Check sheet for the modelled part. Datum: model origin and axes. Units: mm. Face numbers are marked on the shaded views. A direction names the side the tool comes from. Give positions to 0.01 mm unless a question says otherwise; leave off trailing zeros. Write each loop counter-clockwise with the first axis right and the second up, starting at its lowest first coordinate (ties: lowest second). Pieces come first, ordered by that corner, then holes. Notation, with made-up numbers: M 61,-2 L 102,-2 A23 cw 102,32 Z; hole C 45.5,21.25 d7. An arc over 180 degrees is marked long. Write each question's results on one line, items separated by ' | '. Start each with the question number.
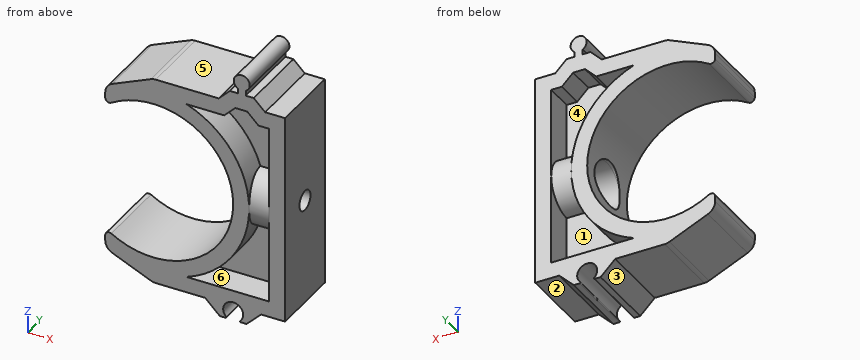
from build123d import *

# Parameters (mm, degrees)
BOSS_EXTRUDE1_DEPTH = 18
CUT_EXTRUDE1_DEPTH  = 7
BOSS_EXTRUDE2_DEPTH = 7
SKETCH4_R           = 2.5
CUT_EXTRUDE2_DEPTH  = 6
SKETCH5_R           = 5.75
CUT_EXTRUDE3_DEPTH  = 7
CUT_EXTRUDE4_START  = -7
SKETCH6_R           = 5.75
CUT_EXTRUDE4_DEPTH  = 7


with BuildPart() as part:
    # Sketch1 → Boss-Extrude1 (new body)
    with BuildSketch(Plane(origin=(0, 0, 0), x_dir=(1, 0, 0), z_dir=(0, 1, 0))):
        with BuildLine():
            Line((10.653013329, -29.309744988), (10.653013329, -30.57769418))
            ThreePointArc((10.653013329, -30.57769418), (11.653013329, -34.309744988), (12.653013329, -30.57769418))
            Line((12.653013329, -30.57769418), (12.653013329, -29.309744988))
            Line((12.653013329, -29.309744988), (14.653013329, -29.309744988))
            Line((14.653013329, -29.309744988), (17.5, -26.5))
            Line((17.5, -26.5), (22.5, -26.5))
            Line((22.5, -26.5), (22.5, 26.5))
            Line((22.5, 26.5), (16.5, 26.5))
            Line((16.5, 26.5), (12.844502727, 30.107679392))
            Line((12.844502727, 30.107679392), (11.410696035, 30.107679392))
            ThreePointArc((11.410696035, 30.107679392), (11.225950376, 29.984289062), (11.269162996, 29.766369807))
            ThreePointArc((11.269162996, 29.766369807), (9.5, 25.5), (7.730837004, 29.766369807))
            ThreePointArc((7.730837004, 29.766369807), (7.774049624, 29.984289062), (7.589303965, 30.107679392))
            Line((7.589303965, 30.107679392), (6.155497273, 30.107679392))
            Line((6.155497273, 30.107679392), (2.5, 26.5))
            Line((2.5, 26.5), (-9.870833143, 26.5))
            ThreePointArc((-9.870833143, 26.5), (-10.486603861, 26.436124388), (-11.076152757, 26.247217616))
            Line((-11.076152757, 26.247217616), (-20.702456422, 22.023754373))
            Line((-20.702456422, 22.023754373), (-20.705319614, 22.022498171))
            ThreePointArc((-20.705319614, 22.022498171), (-22.011569115, 20.916018371), (-22.5, 19.275280555))
            Line((-22.5, 19.275280555), (-22.5, 17.88854382))
            ThreePointArc((-22.5, 17.88854382), (-21.987950036, 17.015672259), (-20.976190476, 17.0367084))
            ThreePointArc((-20.976190476, 17.0367084), (9.5, 0), (-20.976190476, -17.0367084))
            ThreePointArc((-20.976190476, -17.0367084), (-21.987950036, -17.015672259), (-22.5, -17.88854382))
            Line((-22.5, -17.88854382), (-22.5, -19.287953276))
            ThreePointArc((-22.5, -19.287953276), (-22.010713993, -20.929999331), (-20.702456502, -22.03642528))
            Line((-20.702456502, -22.03642528), (-11.074921132, -26.248472005))
            ThreePointArc((-11.074921132, -26.248472005), (-10.486705619, -26.43644479), (-9.87246463, -26.5))
            Line((-9.87246463, -26.5), (5.880022863, -26.5))
            Line((5.880022863, -26.5), (8.653013329, -29.309744988))
            Line((8.653013329, -29.309744988), (10.653013329, -29.309744988))
        make_face()
    extrude(amount=BOSS_EXTRUDE1_DEPTH)

    # Sketch2 → Cut-Extrude1 (cut)
    with BuildSketch(Plane.XZ):
        with BuildLine():
            Line((18.5, 22.5), (18.5, -22.5))
            Line((18.5, -22.5), (-2.148353456, -22.5))
            ThreePointArc((-2.148353456, -22.5), (13.5, 0), (-2.148353456, 22.5))
            Line((-2.148353456, 22.5), (7.238559187, 22.5))
            Line((7.238559187, 22.5), (10.039345887, 25.282038261))
            Line((10.039345887, 25.282038261), (13.039345883, 25.282178795))
            Line((13.039345883, 25.282178795), (15.843268341, 22.5))
            Line((15.843268341, 22.5), (18.5, 22.5))
        make_face()
    cut_extrude1 = extrude(amount=-CUT_EXTRUDE1_DEPTH, mode=Mode.SUBTRACT)

    # Mirror1: Cut-Extrude1 across plane
    add(cut_extrude1.mirror(Plane(origin=(0, 9, 0), x_dir=(0, 0, 1), z_dir=(0, -1, 0))), mode=Mode.SUBTRACT)

    # Sketch3 → Boss-Extrude2 (add)
    with BuildSketch(Plane.ZY.offset(-18.5)):
        with BuildLine():
            Line((7, 7), (-7, 7))
            ThreePointArc((-7, 7), (0, 0), (7, 7))
        make_face()
    boss_extrude2 = extrude(amount=BOSS_EXTRUDE2_DEPTH)

    # Mirror2: Boss-Extrude2 across plane
    add(boss_extrude2.mirror(Plane(origin=(0, 9, 0), x_dir=(0, 0, 1), z_dir=(0, -1, 0))))

    # Sketch4 → Cut-Extrude2 (cut)
    with BuildSketch(Plane(origin=(22.5, 0, 0), x_dir=(0, 0, -1), z_dir=(1, 0, 0))):
        with Locations((0, 9)):
            Circle(SKETCH4_R)
    extrude(amount=-CUT_EXTRUDE2_DEPTH, mode=Mode.SUBTRACT)

    # Sketch5 → Cut-Extrude3 (cut)
    with BuildSketch(Plane(origin=(9.5, 0, 0), x_dir=(0, 0, -1), z_dir=(1, 0, 0))):
        with Locations((0, 9)):
            Circle(SKETCH5_R)
    extrude(amount=-CUT_EXTRUDE3_DEPTH, mode=Mode.SUBTRACT)

    # Sketch6 → Cut-Extrude4 (cut)
    with BuildSketch(Plane.ZY.offset(-9.5).offset(CUT_EXTRUDE4_START)):
        with Locations(Location((0, 9, 0), (0, 0, 180))):
            Circle(SKETCH6_R)
    extrude(amount=CUT_EXTRUDE4_DEPTH, mode=Mode.SUBTRACT)


solid = part.part
Q1. Tool access check on the marked faces 4, 5 and 6. Record the directions out of +Z, -Z, +X, -X, +Y, -Y that give a thin tool (end or side, any length) a straight path to the whole face; none if there is none.
Q2. Scan lines: L1, parallel to Z at x = 10.5, y = 7.5; L2, parallel to Z at x = 10, y = 14; L3, parallel to Z at x = 6, y = 13.5. Record each from-to range of solid material in increasing order.
Q3. Depth check by flat-ended pin: pin 1 Ø4 at (x, y) = (2, 10.5) entering from -Z; pin 2 Ø2 at (y, z) = (6.5, -5.5) entering from -X; pin 3 Ø2 at (x, y) = (17, 4) entering from -Z. Enter the tip coordinate at first touch or a pass-through.
Q4. Section check A-A on x = 1. Record the boundary of the cut face in (y, z), plus the area to 3 significant figures.
Q5. Section check D-D on z = 10. Record the boundary of the cut face in (x, y), plus the area to 3 significant figures.
Q6. Release check for a two-part mould opening along X. For the marked faces 1, 2 and 3 record: pulls with the +X half, pulls with the -X half, needs draft (parallel to the pull), parting line crosses it, or undercut.
Q7. Section check C-C on y = 16. State how many separate pieces and enclosed holes the cut face has, plus the area to 3 significant figures.
Q8. Section check B-B on z = -12. Record the boundary of the cut face in (x, y), plus the area to 3 significant figures.
Check result:
1) face 4: +Y | face 5: +Z, -X, +Y, -Y | face 6: -Y
2) L1: -25.71 to -5.55, 5.55 to 29.31, 30.68 to 33.94 | L2: -25.55 to -22.5, -12.48 to -2.84, 2.84 to 12.48, 25.24 to 29.31, 31.18 to 33.44 | L3: -29.95 to -22.5, -17.43 to -11.3, 11.3 to 17.43, 22.5 to 26.62
3) pin 1: z = -27.98 | pin 2: x = 8.41 | pin 3: z = -26.99
4) outline: M 0,-26.5 L 18,-26.5 L 18,-22.5 L 11,-22.5 L 11,-21.07 L 18,-21.07 L 18,-16.36 L 0,-16.36 L 0,-21.07 L 7,-21.07 L 7,-22.5 L 0,-22.5 Z; M 0,16.36 L 18,16.36 L 18,21.07 L 11,21.07 L 11,22.5 L 18,22.5 L 18,26.5 L 0,26.5 L 0,22.5 L 7,22.5 L 7,21.07 L 0,21.07 Z | area: 325 mm^2
5) outline: M 6.82,0 L 11.32,0 L 11.32,7 L 18.5,7 L 18.5,0 L 22.5,0 L 22.5,18 L 18.5,18 L 18.5,11 L 11.32,11 L 11.32,18 L 6.82,18 Z | area: 182 mm^2
6) face 1: undercut | face 2: needs draft | face 3: pulls with the -X half
7) separate pieces: 1 | enclosed holes: 2 | area: 916 mm^2
8) outline: M 5.5,0 L 10.28,0 L 10.28,7 L 18.5,7 L 18.5,0 L 22.5,0 L 22.5,18 L 18.5,18 L 18.5,11 L 10.28,11 L 10.28,18 L 5.5,18 Z | area: 191 mm^2
